```python
from build123d import *

# Parameters (mm, degrees)
F1_DEPTH = 180
F2_DEPTH = 3


with BuildPart() as f1:
    # F0 (on Top) → F1 (new body)
    with BuildSketch(Plane.XY):
        with BuildLine():
            ThreePointArc((-54.459718, -40.720255), (-64.038422, -21.381102), (-66.971492, 0))
            Line((-66.971492, 0), (-68, 0))
            ThreePointArc((-68, 0), (-64.526199, -21.456225), (-54.459718, -40.720255))
        make_face()
        with BuildLine():
            Line((-68, 0), (-66.971492, 0))
            ThreePointArc((-66.971492, 0), (0.852343, 65.28321), (66.99318, -1.704548))
            ThreePointArc((66.99318, -1.704548), (63.782897, -22.194259), (54.459718, -40.720255))
            ThreePointArc((54.459718, -40.720255), (64.526199, -21.456225), (68, 0))
            ThreePointArc((68, 0), (0, 68), (-68, 0))
        make_face()
        with BuildLine():
            ThreePointArc((65, 0), (0, 65), (-65, 0))
            ThreePointArc((-65, 0), (0, -65), (65, 0))
        make_face()
        with BuildLine():
            ThreePointArc((54.459718, -40.720255), (0, -68), (-54.459718, -40.720255))
            ThreePointArc((-54.459718, -40.720255), (0, -68.697729), (54.459718, -40.720255))
        make_face()
        with BuildLine():
            ThreePointArc((66.99318, -1.704548), (0.852343, 65.28321), (-66.971492, 0))
            ThreePointArc((-66.971492, 0), (-64.038422, -21.381102), (-54.459718, -40.720255))
            ThreePointArc((-54.459718, -40.720255), (0, -68), (54.459718, -40.720255))
            ThreePointArc((54.459718, -40.720255), (63.782897, -22.194259), (66.99318, -1.704548))
        make_face()
        with BuildLine():
            ThreePointArc((65, 0), (0, -65), (-65, 0))
            ThreePointArc((-65, 0), (0, 65), (65, 0))
        make_face(mode=Mode.SUBTRACT)
    extrude(amount=F1_DEPTH)

    # F0 (on Top) → F2 (join)
    with BuildSketch(Plane.XY):
        with BuildLine():
            ThreePointArc((65, 0), (0, 65), (-65, 0))
            ThreePointArc((-65, 0), (0, -65), (65, 0))
        make_face()
    extrude(amount=F2_DEPTH)


solid = f1.part
```
Can you work these out from the model? Positions are in its coordinate system, mm. A direction names the side the tool comes from. Coordinates: 2 decimals unless noted, no trailing zeros. Loops run counter-clockwise (first coordinate to the right, second up) from the corner with the lowest first, then second, coordinate; pieces in that order, holes last.
1) Thinking about a two-plate mould opening in Y: for faces 1 (the cylindrical face through (1.495, 67.984, 88.74)), 2 (the flat face through (-1, 1, 0)), 3 (the cylindrical face through (-62, 19.52, 90.26)), 4 (the cylindrical face through (-64.62, -21.17, 88.74)), which applies, pulls with the +Y half, pulls with the -Y half, needs draft (parallel to the pull), parting line crosses it, or undercut?
2) I need wall thicknesses on probe 1 along Y at (x, z) = (0, 116); probe 2 along Z at (x, y) = (24, 50); probe 3 along X at (y, z) = (-38.5, 135). Which ranges of each line are inside material? Lowest first, please.
3) Imagine slicing it at C-C on y = -58. List the corners of the cut face in (x, z) for me, plus the area to 3 significant figures.
4) Imagine slicing it at B-B on z = 76.5. List the corners of the cut face in (x, y) for me.
5) For pin 1 (8 mm diameter, centred on y = 8, z = 36.5, fed in from -X); pin 2 (4 mm diameter, centred on y = -54.5, z = 96, fed in from -X); pin 3 (1 mm diameter, centred on x = -6.5, z = 84, fed in from -Y), each with a flat end and sliding along its axis, tell me the tip position at first contact or that it passes through.
6) Imagine slicing it at A-A on x = 0. List the corners of the cut face in (y, z) for me, plus the area to 3 significant figures.
7) Which directions (+Z, -Z, +X, -X, +Y, -Y) give clear straight access to the entire face, cutting with the end or side of a thin tool? Please do faces 5 (the cylindrical face through (-0.89, -68.69, 88.74)), 6 (the flat face through (-1, 1, 3)).
Completed:
1. face 1: pulls with the +Y half
1. face 2: needs draft
1. face 3: undercut
1. face 4: pulls with the -Y half
2. probe 1: y = -68.7 to -65, 65 to 68
2. probe 2: z = 0 to 3
2. probe 3: x = -56.05 to -52.37, 52.37 to 56.05
3. outline: (-36.32, 0) - (36.32, 0) - (36.32, 180) - (29.34, 180) - (29.34, 3) - (-29.34, 3) - (-29.34, 180) - (-36.32, 180) - close
3. area: 2,690 mm2
4. outline: (-68, 0) arc R68 ccw to (-54.46, -40.72) arc R66.99 ccw to (54.46, -40.72) arc R68 ccw to (68, 0) arc R68 ccw to start; hole circle Ø130 at (0, 0)
5. pin 1: stops at x = -67.88
5. pin 2: stops at x = -43.68
5. pin 3: stops at y = -68.43
6. outline: (-68.7, 0) - (68, 0) - (68, 180) - (65, 180) - (65, 3) - (-65, 3) - (-65, 180) - (-68.7, 180) - close
6. area: 1,600 mm2
7. face 5: +Z, -Z, -Y
7. face 6: +Z
